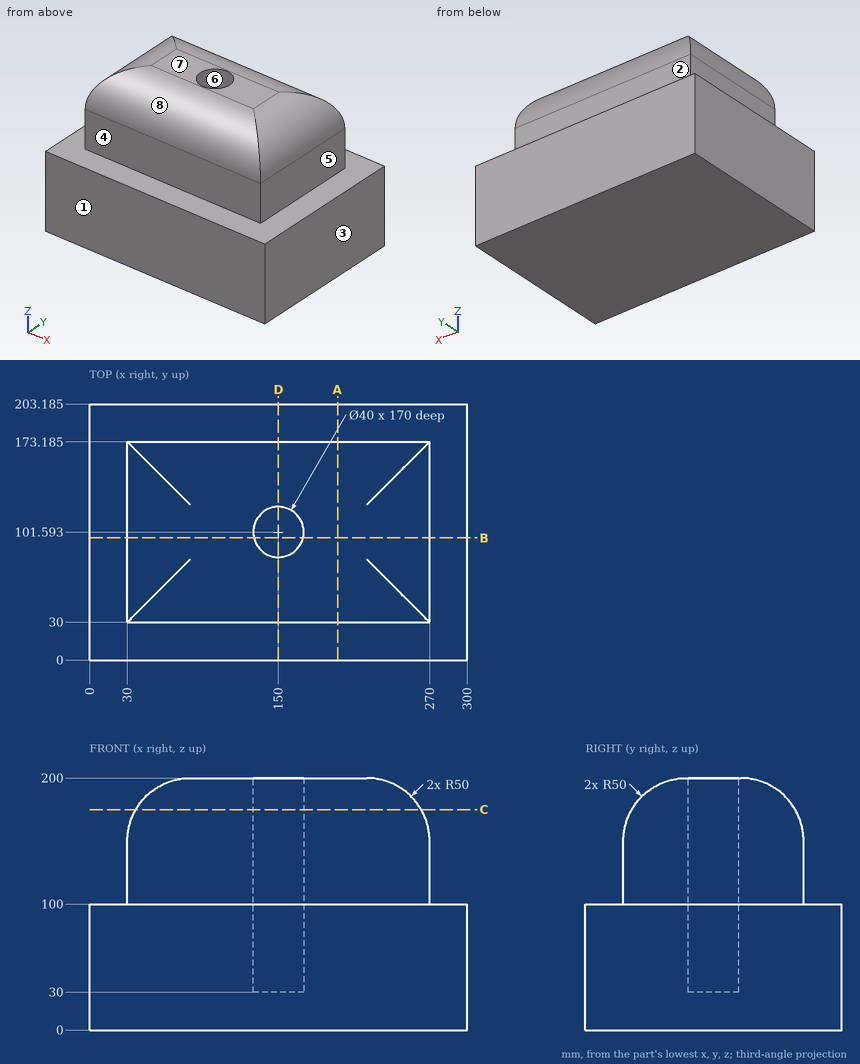
For this review, use the dimensioned drawing (mm, ordinates from the lowest corner) and the shaded views. A direction names the side the tool comes from. Round coordinates to 2 decimals unless told otherwise and drop trailing zeros. Write each loop counter-clockwise with the first axis right and the second up, starting at its lowest first coordinate (ties: lowest second). Pieces come first, ordered by that corner, then holes. Notation, with made-up numbers: (-27.5, -32.75) - (20.5, -32.75) arc R21 cw to (20.5, -6.75) - close; hole circle Ø8 at (-1.75, 33.25). An arc over 180 degrees is marked (long way). Answer as CSV lines item,"result". Start each with the question number.
(1) We need section D-D on x = 150. State the section outline as (y, z) points (1 decimal), plus the area to 3 significant figures.
(2) We need section B-B on y = 97. State the section outline as (x, z) points (1 decimal), plus the area to 3 significant figures.
(3) To check wall thickness, follow line 1 (Y direction, x = 150, z = 132.5) (1 decimal); line 2 (Y direction, x = 150, z = 71) (1 decimal); line 3 (Z direction, x = 189, y = 177.5). State the ranges of each line that lie inside material, in increasing order.
(4) For the marked faces 1, 2, 3, 4 and 5, list the 3-axis set-ups (+Z, -Z, +X, -X, +Y, -Y) from which the entire face can be reached by the end or side of a thin tool; tool diameter is ignored.
(5) We need section C-C on z = 175. State the section outline as (x, y) points.
(6) For pin 1 Ø2 at (y, z) = (101.5, 166) entering from -X; pin 2 Ø2 at (x, y) = (220, 44.5) entering from +Z; pin 3 Ø25 at (x, z) = (129, 120.5) entering from +Y (1 decimal), all flat-tipped, find the tip position at first contact; note any pin that passes through.
(7) We need section A-A on x = 197. State the section outline as (y, z) points (1 decimal), plus the area to 3 significant figures.
(8) Draft analysis for pull direction Y (two halves, no side actions). For the marked faces 6, 7 and 8, state which applies: pulls with the +Y half, pulls with the -Y half, needs draft (parallel to the pull), parting line crosses it, or undercut.
Worked answers:
1,outline,"(0, 0) - (203.2, 0) - (203.2, 100) - (173.2, 100) - (173.2, 150) arc R50 ccw to (123.2, 200) - (121.6, 200) - (121.6, 30) - (81.6, 30) - (81.6, 200) - (80, 200) arc R50 ccw to (30, 150) - (30, 100) - (0, 100) - close"
1,area,"26,800 mm²"
2,outline,"(0, 0) - (300, 0) - (300, 100) - (270, 100) - (270, 150) arc R50 ccw to (220, 200) - (169.5, 200) - (169.5, 30) - (130.5, 30) - (130.5, 200) - (80, 200) arc R50 ccw to (30, 150) - (30, 100) - (0, 100) - close"
2,area,"46,300 mm²"
3,line 1,"30 to 81.6, 121.6 to 173.2"
3,line 2,"0 to 81.6, 121.6 to 203.2"
3,line 3,"0 to 100"
4,face 1,"+Z, -Z, +X, -X, -Y"
4,face 2,"+Z, +X, -X, +Y"
4,face 3,"+Z, -Z, +X, +Y, -Y"
4,face 4,"+Z, +X, -X, -Y"
4,face 5,"+Z, +X, +Y, -Y"
5,outline,"(36.7, 36.7) - (263.3, 36.7) - (263.3, 166.49) - (36.7, 166.49) - close; hole circle Ø40 at (150, 101.59)"
6,pin 1,"x = 32.3"
6,pin 2,"z = 186.19"
6,pin 3,"y = 173.2"
7,outline,"(0, 0) - (203.2, 0) - (203.2, 100) - (173.2, 100) - (173.2, 150) arc R50 ccw to (123.2, 200) - (80, 200) arc R50 ccw to (30, 150) - (30, 100) - (0, 100) - close"
7,area,"33,600 mm²"
8,face 6,"undercut"
8,face 7,"needs draft"
8,face 8,"pulls with the -Y half"
